from build123d import *

# Parameters (mm, degrees)
ESQUISSE2_W             = 8
ESQUISSE2_H             = 8
ENL_V_MAT_EXTRU_1_DEPTH = 13.5
ESQUISSE3_R             = 6
ENL_V_MAT_EXTRU_2_DEPTH = 10
ESQUISSE4_R             = 3
ENL_V_MAT_EXTRU_3_DEPTH = 10


with BuildPart() as part:
    # Esquisse1 → Révolution1 (revolve)
    with BuildSketch(Plane.XY):
        Polygon((0, 0), (0, 8.5), (3, 8.5), (3, 9.093663992), (3, 10), (5, 10), (5, 7.5), (12.5, 7.5), (12.5, 0), align=None)
    revolve(axis=Axis((-59.603539616, 0, 0), (1, 0, 0)))

    # Esquisse2 → Enlèv. mat.-Extru.1 (cut, through all)
    with BuildSketch(Plane.ZY):
        Rectangle(ESQUISSE2_W, ESQUISSE2_H)
    extrude(amount=-ENL_V_MAT_EXTRU_1_DEPTH, mode=Mode.SUBTRACT)

    # Esquisse3 → Enlèv. mat.-Extru.2 (cut)
    with BuildSketch(Plane(origin=(12.5, 0, 0), x_dir=(0, 0, -1), z_dir=(1, 0, 0))):
        Circle(ESQUISSE3_R)
    extrude(amount=-ENL_V_MAT_EXTRU_2_DEPTH, mode=Mode.SUBTRACT)

    # Esquisse4 → Enlèv. mat.-Extru.3 (cut)
    with BuildSketch(Plane(origin=(0, 0, 0), x_dir=(1, 0, 0), z_dir=(0, 1, 0))):
        with Locations((8.5, 0)):
            Circle(ESQUISSE4_R)
    extrude(amount=-ENL_V_MAT_EXTRU_3_DEPTH, mode=Mode.SUBTRACT)


solid = part.part
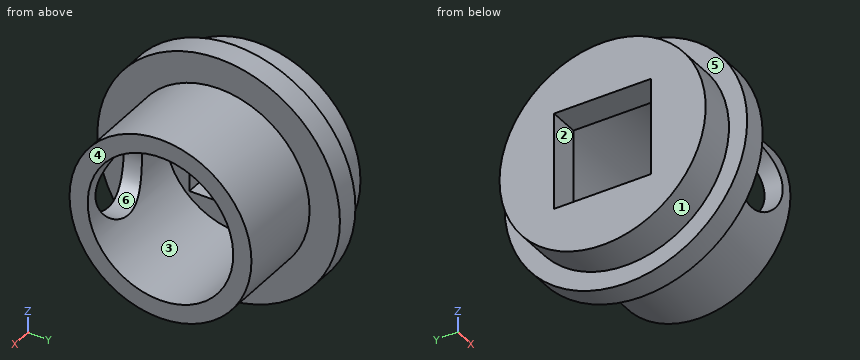
Part model, mm, in its own coordinate system. Face numbers are marked on the shaded views. A direction names the side the tool comes from. Coordinates: 2 decimals unless noted, no trailing zeros. Order: outer loops, then holes, each group sorted by start corner. A loop starts at its lowest first (then second) coordinate and runs counter-clockwise, first axis right, second up.
(1) Probe L1, parallel to X at y = -6.55, z = 0; L2, parallel to X at y = 1.75, z = -8.5; L3, parallel to X at y = 7.75, z = 0. List the from-to ranges inside material, lowest first.
Check sheet entries:
L1: x = 0 to 5.5, 11.5 to 12.5
L2: x = 3 to 5
L3: x = 0 to 5
(2) Slice it at C-C, the plane x = 5.25. Write the cut outline in (y, z), and give its area (3 significant figures).
Check sheet entries:
outline: circle Ø15 at (0, 0); hole circle Ø12 at (0, 0)
area: 63.6 mm2
(3) Pull direction X, two halves, no side cores. Call the marked faces 4, 5 and 6: pulls with the +X half, pulls with the -X half, needs draft (parallel to the pull), parting line crosses it, or undercut.
Check sheet entries:
face 4: pulls with the +X half
face 5: pulls with the -X half
face 6: undercut
(4) Tool access for the marked faces 1, 2 and 3: list every direction of +Z, -Z, +X, -X, +Y, -Y with a clear straight run to the whole face (end or side of a thin tool).
Check sheet entries:
face 1: -X
face 2: +X, -X
face 3: +X
(5) Slice it at B-B, the plane z = 0. Write the cut outline in (x, y).
Check sheet entries:
outline: (0, -8.5) - (3, -8.5) - (3, -10) - (5, -10) - (5, -7.5) - (5.5, -7.5) - (5.5, -6) - (2.5, -6) - (2.5, -4) - (0, -4) - close; (0, 4) - (2.5, 4) - (2.5, 6) - (12.5, 6) - (12.5, 7.5) - (5, 7.5) - (5, 10) - (3, 10) - (3, 8.5) - (0, 8.5) - close; (11.5, -7.5) - (12.5, -7.5) - (12.5, -6) - (11.5, -6) - close
(6) Slice it at D-D, the plane z = -6.5. Write the cut outline in (x, y).
Check sheet entries:
outline: (0, -5.48) - (3, -5.48) - (3, -7.6) - (5, -7.6) - (5, -3.74) - (12.5, -3.74) - (12.5, 3.74) - (5, 3.74) - (5, 7.6) - (3, 7.6) - (3, 5.48) - (0, 5.48) - close
(7) Pin check, flat tips, straight feed: pin 1 Ø1 at (y, z) = (7.5, 7) entering from +X; pin 2 Ø3 at (x, z) = (0.5, 1.5) entering from +Y; pin 3 Ø1.2 at (x, y) = (1, -1) entering from +Z. Stop position of each tip, or through.
Check sheet entries:
pin 1: stops at x = 5
pin 2: stops at y = 8.5
pin 3: stops at z = 8.49
(8) Slice it at A-A, the plane y = 0. Write the cut outline in (x, z).
Check sheet entries:
outline: (0, -8.5) - (3, -8.5) - (3, -10) - (5, -10) - (5, -7.5) - (12.5, -7.5) - (12.5, -6) - (2.5, -6) - (2.5, -4) - (0, -4) - close; (0, 4) - (2.5, 4) - (2.5, 6) - (12.5, 6) - (12.5, 7.5) - (5, 7.5) - (5, 10) - (3, 10) - (3, 8.5) - (0, 8.5) - close
